Here's how the part is built. I have some questions about the finished solid (model axes, mm). A direction names the side the tool comes from. Coordinates: 2 decimals unless noted, no trailing zeros. Write each loop counter-clockwise with the first axis right and the second up, starting at its lowest first coordinate (ties: lowest second). Pieces come first, ordered by that corner, then holes. Notation, with made-up numbers: (73, 40) -> (125, 40) arc R12 ccw to (125, 62) -> close; hole circle Ø6 at (-11, -7). An arc over 180 degrees is marked (long way). Put each result on its own line as item: value. Start each with the question number.
Item 1: I want a section at B-B, the plane x = -23228. List the corners of the cut face in (y, z) for me.
Item 2: I want a section at D-D, the plane z = 40742. List the corners of the cut face in (x, y) for me.
Item 3: For pin 1 (3 mm diameter, centred on y = 6084.5, z = 40838, fed in from +X); pin 2 (6 mm diameter, centred on y = 6075, z = 40306, fed in from +X), each with a flat end and sliding along its axis, tell me the tip position at first contact or that it passes through.
Item 4: If we mould it in two halves opening along Z, with no side actions, what happens to faces 4 (the face through (-23177, 6067.857, 40544)), 5 (the face through (-23098, 6078, 41050.141)), 6 (the face through (-23057, 6078, 40189.1)), 7 (the face through (-23163, 6078, 40022.681))? For each: released by +Z, released by -Z, zero draft, split by the parting line, or undercut.
Item 5: I want a section at A-A, the plane x = -23135.5. List the corners of the cut face in (y, z) for me.
Item 6: I need wall thicknesses on line 1 (Z direction, x = -23156.5, y = 6083); line 2 (Z direction, x = -22854.5, y = 6069); line 3 (Z direction, x = -23231, y = 6078.75). Which ranges of each line are inside material? Lowest first, please. Write a range as [from, to].
Item 7: On a 3-axis mill with a long thin cutter (end or side, diameter ignored), from which of +Z, -Z, +X, -X, +Y, -Y can I reach the whole of each face in a straight line? I mean faces 1 (the face through (-22786.083, 6078, 40521)), 2 (the face through (-23004, 6078, 40447.925)), 3 (the face through (-22901.561, 6078, 40105)). Say none if no direction works.
Item 8: I want a section at C-C, the plane y = 6082.5. List the corners of the cut face in (x, z) for me.
from build123d import *

# Parameters (mm, degrees)
BOSS_EXTRUDE1_START = 500
BOSS_EXTRUDE1_DEPTH = 20


with BuildPart() as part:
    # Sketch2 → Boss-Extrude1 (new body)
    with BuildSketch(Plane.XZ.offset(-6587.857128547).offset(BOSS_EXTRUDE1_START)):
        Polygon((-23417.771071287, 41050.141416955), (-23417.771071287, 40189.100196056), (-23417.771071287, 40022.680514279), (-22901.561141737, 40022.680514279), (-22901.561141737, 40189.100196056), (-23216.614310756, 40189.100196056), (-23216.614310756, 40447.924756229), (-22786.083114137, 40447.924756229), (-22786.083114137, 40595.178045331), (-23241.381102723, 40595.178045331), (-23241.381102723, 40904.737128326), (-22786.083114137, 40904.737128326), (-22786.083114137, 41050.141416955), align=None)
    extrude(amount=BOSS_EXTRUDE1_DEPTH)


solid = part.part
Calculated:
1. outline: (6067.86, 40022.68) -> (6087.86, 40022.68) -> (6087.86, 40595.18) -> (6067.86, 40595.18) -> close; (6067.86, 40904.74) -> (6087.86, 40904.74) -> (6087.86, 41050.14) -> (6067.86, 41050.14) -> close
2. outline: (-23417.77, 6067.86) -> (-23241.38, 6067.86) -> (-23241.38, 6087.86) -> (-23417.77, 6087.86) -> close
3. pin 1: stops at x = -23241.38
3. pin 2: stops at x = -23216.61
4. face 4: zero draft
4. face 5: released by +Z
4. face 6: undercut
4. face 7: released by -Z
5. outline: (6067.86, 40022.68) -> (6087.86, 40022.68) -> (6087.86, 40189.1) -> (6067.86, 40189.1) -> close; (6067.86, 40447.92) -> (6087.86, 40447.92) -> (6087.86, 40595.18) -> (6067.86, 40595.18) -> close; (6067.86, 40904.74) -> (6087.86, 40904.74) -> (6087.86, 41050.14) -> (6067.86, 41050.14) -> close
6. line 1: z = [40022.68, 40189.1], [40447.92, 40595.18], [40904.74, 41050.14]
6. line 2: z = [40447.92, 40595.18], [40904.74, 41050.14]
6. line 3: z = [40022.68, 40595.18], [40904.74, 41050.14]
7. face 1: +Z, -Z, +X, +Y, -Y
7. face 2: +X, +Y, -Y
7. face 3: -Z, +X, +Y, -Y
8. outline: (-23417.77, 40022.68) -> (-22901.56, 40022.68) -> (-22901.56, 40189.1) -> (-23216.61, 40189.1) -> (-23216.61, 40447.92) -> (-22786.08, 40447.92) -> (-22786.08, 40595.18) -> (-23241.38, 40595.18) -> (-23241.38, 40904.74) -> (-22786.08, 40904.74) -> (-22786.08, 41050.14) -> (-23417.77, 41050.14) -> close
